Work out the finished part from the listing and answer in its coordinate system (mm). Give positions to 0.01 mm unless a question says otherwise; leave off trailing zeros. Order: outer loops, then holes, each group sorted by start corner. A loop starts at its lowest first (then second) coordinate and runs counter-clockwise, first axis right, second up.
```python
from build123d import *

# Parameters (mm, degrees)
SKETCH_1_R      = 1.5
SKETCH_1_R_2    = 2
SKETCH_1_R_3    = 5
EXTRUDE_1_DEPTH = 2


with BuildPart() as part:
    # Эскиз1 → Бобышка-Вытянуть1 (new body)
    with BuildSketch(Plane(origin=(0, 0, 0), x_dir=(1, 0, 0), z_dir=(0, 1, 0))):
        with BuildLine():
            Line((12.374772085, -29.617278809), (12.374772085, 20.682721191))
            Line((12.374772085, 20.682721191), (9.374772085, 39.182721191))
            ThreePointArc((9.374772085, 39.182721191), (-2.625227915, 51.182721191), (-14.625227915, 39.182721191))
            Line((-14.625227915, 39.182721191), (-17.625227915, 20.682721191))
            Line((-17.625227915, 20.682721191), (-17.625227915, -29.617278809))
            Line((-17.625227915, -29.617278809), (-10.625227915, -29.617278809))
            Line((-10.625227915, -29.617278809), (5.374772085, -29.617278809))
            Line((5.374772085, -29.617278809), (12.374772085, -29.617278809))
        make_face()
        with Locations(Location((-13.625227915, -26.117278809, 0), (0, 0, 270))):
            Circle(SKETCH_1_R, mode=Mode.SUBTRACT)
        with Locations(Location((8.374772085, -26.117278809, 0), (0, 0, 270))):
            Circle(SKETCH_1_R, mode=Mode.SUBTRACT)
        with Locations(Location((-2.625227915, 39.182721191, 0), (0, 0, 270))):
            Circle(SKETCH_1_R_2, mode=Mode.SUBTRACT)
        with Locations(Location((-2.625227915, 1.972721191, 0), (0, 0, 270))):
            Circle(SKETCH_1_R_3, mode=Mode.SUBTRACT)
    extrude(amount=EXTRUDE_1_DEPTH)


solid = part.part
```
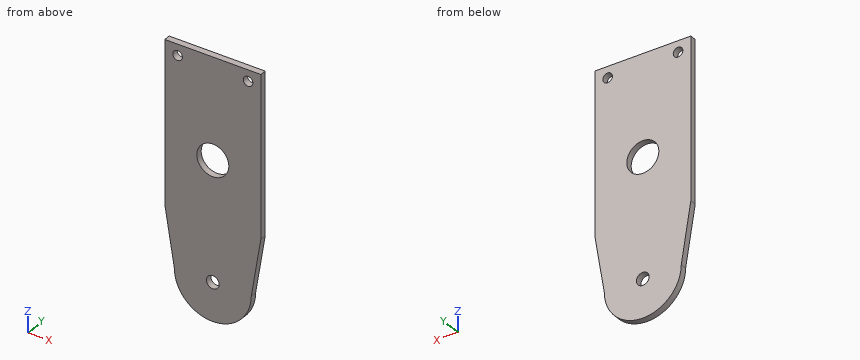
1. Given P1, Ø5, axis at x = -2.63, z = -39.18, coming from the -Y side; P2, Ø9, axis at x = -2.63, z = -1.97, coming from the +Y side, each flat-ended and moving along its own axis, determine where each tip first touches the part or whether it passes through.
Findings below:
P1: stops at y = 0
P2: passes through
2. Straight lines are drawn through the part: probe 1 along Z at (x, y) = (-2.5, 1.5); probe 2 along Z at (x, y) = (-3, 1.4); probe 3 along Z at (x, y) = (-13.5, 0.85). For each, find the intervals that lie inside material, in ascending order.
Findings below:
probe 1: z = -51.18 to -41.18, -37.19 to -6.97, 3.03 to 29.62
probe 2: z = -51.18 to -41.15, -37.22 to -6.96, 3.01 to 29.62
probe 3: z = -44.26 to 24.62, 27.61 to 29.62
3. The part is cut by section C-C (z = -44). Write down the section's boundary in (x, y).
Findings below:
outline: (-13.62, 0) - (8.37, 0) - (8.37, 2) - (-13.62, 2) - close
4. The part is cut by section A-A (y = 1.05). Write down the section's boundary in (x, z).
Findings below:
outline: (-17.63, -20.68) - (-14.63, -39.18) arc R12 ccw to (9.37, -39.18) - (12.37, -20.68) - (12.37, 29.62) - (-17.63, 29.62) - close; hole circle Ø3 at (-13.63, 26.12); hole circle Ø10 at (-2.63, -1.97); hole circle Ø4 at (-2.63, -39.18); hole circle Ø3 at (8.37, 26.12)
5. The part is cut by section B-B (x = 4.5). Write down the section's boundary in (y, z).
Findings below:
outline: (0, -48.84) - (2, -48.84) - (2, 29.62) - (0, 29.62) - close
